Can you work these out from the model? Positions are in its coordinate system, mm. A direction names the side the tool comes from. Give positions to 0.01 mm unless a question says otherwise; leave off trailing zeros. Loops run counter-clockwise (first coordinate to the right, second up) from the corner with the lowest first, then second, coordinate; pieces in that order, holes last. Notation, with made-up numbers: M 78.5,24.25 L 114.5,24.25 A12 ccw 114.5,45.25 Z; hole C 64,-10.75 d9. An arc over 180 degrees is marked long. Answer as a JSON object with one key per item and string values.
```python
from build123d import *

# Parameters (mm, degrees)
SKETCH1_W           = 60
SKETCH1_H           = 30
SKETCH1_R           = 7.5
BOSS_EXTRUDE1_DEPTH = 25
SKETCH2_R           = 2.5
CUT_EXTRUDE1_DEPTH  = 30


with BuildPart() as part:
    # Sketch1 → Boss-Extrude1 (new body, symmetric)
    with BuildSketch(Plane.XY):
        with Locations((250, 0)):
            Rectangle(SKETCH1_W, SKETCH1_H)
        with Locations((250, 0)):
            Circle(SKETCH1_R, mode=Mode.SUBTRACT)
    extrude(amount=BOSS_EXTRUDE1_DEPTH, both=True)

    # Sketch2 → Cut-Extrude1 (cut)
    with BuildSketch(Plane.ZY.offset(-220)):
        with Locations((13.5, 0)):
            Circle(SKETCH2_R)
        with Locations((-13.5, 0)):
            Circle(SKETCH2_R)
    extrude(amount=-CUT_EXTRUDE1_DEPTH, mode=Mode.SUBTRACT)


solid = part.part
```
1) If we mould it in two halves opening along Z, with no side actions, what happens to faces 1 (the flat face through (250, 15, 0)), 2 (the cylindrical face through (231, 0, 11)), 3 (the flat face through (243, 4, 25))? For each: +Z half, -Z half, draft (parallel to the pull), parting line (faces both ways), or undercut.
Answer list:
{"face 1": "draft", "face 2": "undercut", "face 3": "+Z half"}
2) Suppose I cut it at C-C, the plane x = 250. Write out the boundary of the cut face in (y, z).
Answer list:
{"outline": "M -15,-25 L -7.5,-25 L -7.5,25 L -15,25 Z; M 7.5,-25 L 15,-25 L 15,25 L 7.5,25 Z"}
3) Suppose I cut it at A-A, the plane y = 0. Write out the boundary of the cut face in (x, z), and give its area (4 significant figures).
Answer list:
{"outline": "M 220,-25 L 242.5,-25 L 242.5,-16 L 220,-16 Z; M 220,-11 L 242.5,-11 L 242.5,11 L 220,11 Z; M 220,16 L 242.5,16 L 242.5,25 L 220,25 Z; M 257.5,-25 L 280,-25 L 280,25 L 257.5,25 Z", "area": "2,025 mm^2"}
4) Please list where these lines run through material, in increasing order: line 1 along Z through (x, y) = (229.5, 0); line 2 along Y through (x, z) = (250, 15); line 3 along Y through (x, z) = (226, -13.5). Write a range as from..to.
Answer list:
{"line 1": "-25..-16, -11..11, 16..25", "line 2": "-15..-7.5, 7.5..15", "line 3": "-15..-2.5, 2.5..15"}
5) For faces 4 (the cylindrical face through (231, 0, -16)), 5 (the cylindrical face through (256.93, -2.87, -0.35)), which set-ups out of +Z, -Z, +X, -X, +Y, -Y let a thin tool reach every point of the face, with its end or its side?
Answer list:
{"face 4": "-X", "face 5": "+Z, -Z"}
6) Will this pin go through, and if not, where does the flat tip stop? pin 1 Ø5 at (x, y) = (251.5, -2.5) entering from -Z.
Answer list:
{"pin 1": "through"}
7) Suppose I cut it at D-D, the plane z = 17. Write out the boundary of the cut face in (x, y), and give its area (3 significant figures).
Answer list:
{"outline": "M 220,-15 L 280,-15 L 280,15 L 220,15 Z; hole C 250,0 d15", "area": "1,620 mm^2"}
8) Suppose I cut it at B-B, the plane y = -6. Write out the boundary of the cut face in (x, z).
Answer list:
{"outline": "M 220,-25 L 245.5,-25 L 245.5,25 L 220,25 Z; M 254.5,-25 L 280,-25 L 280,25 L 254.5,25 Z"}
